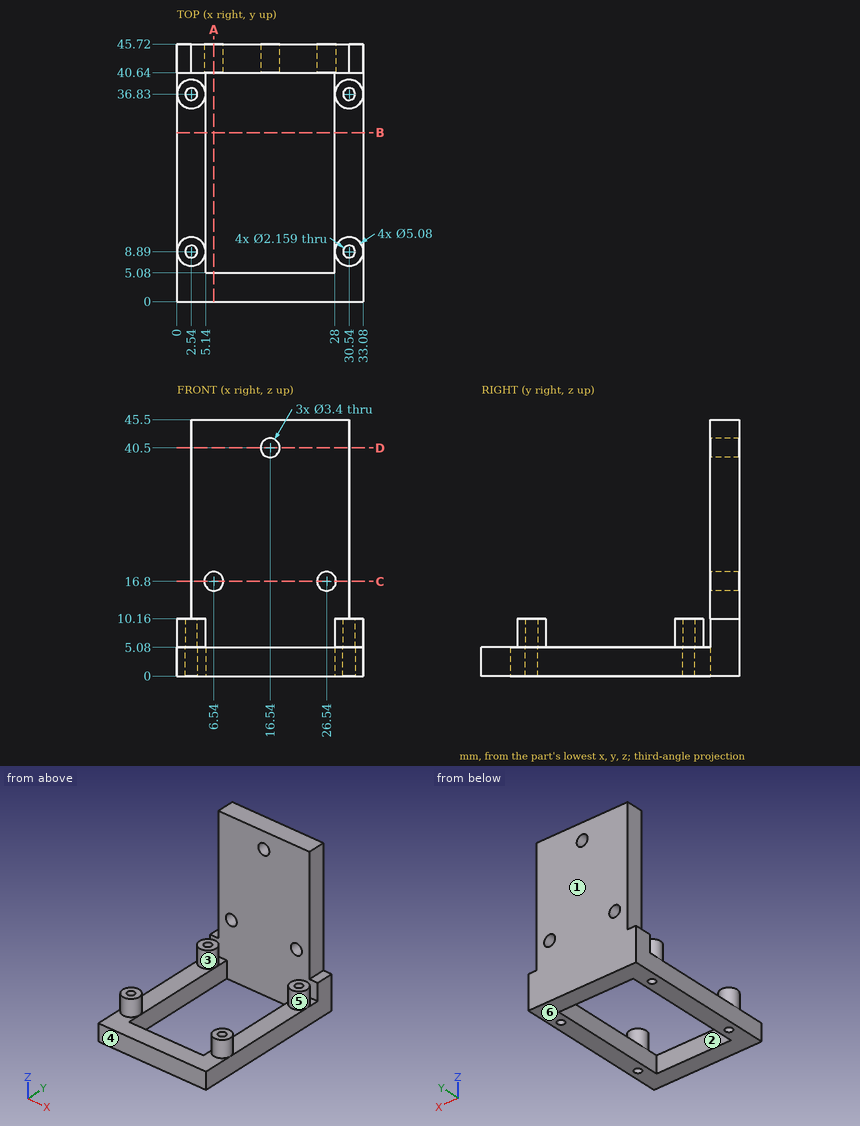
Could you check a few things on this drawing? It's one solid part, dimensions in mm from its lowest x, y, z. A direction names the side the tool comes from. Round coordinates to 2 decimals unless told otherwise and drop trailing zeros. Loops run counter-clockwise (first coordinate to the right, second up) from the corner with the lowest first, then second, coordinate; pieces in that order, holes last. Notation, with made-up numbers: (-24, 86) -> (15, 86) arc R10 ccw to (15, 90) -> close; hole circle Ø7 at (-17.75, -2.5). An arc over 180 degrees is marked (long way). Answer as CSV lines item,"result".
1. If we section it at D-D on z = 40.5: Please give me the cut outline in (x, y), plus the area to 3 significant figures.
Final values:
outline,"(2.54, 40.64) -> (14.84, 40.64) -> (14.84, 45.72) -> (2.54, 45.72) -> close; (18.24, 40.64) -> (30.54, 40.64) -> (30.54, 45.72) -> (18.24, 45.72) -> close"
area,"125 mm^2"
2. Thinking about a two-plate mould opening in Y: for the marked faces 4, 5 and 6, which applies, released by +Y, released by -Y, zero draft, split by the parting line, or undercut?
Final values:
face 4,"released by -Y"
face 5,"undercut"
face 6,"zero draft"
3. If we section it at B-B on y = 30: Please give me the cut outline in (x, z), plus the area to 3 significant figures.
Final values:
outline,"(0, 0) -> (5.14, 0) -> (5.14, 5.08) -> (0, 5.08) -> close; (28, 0) -> (33.08, 0) -> (33.08, 5.08) -> (28, 5.08) -> close"
area,"51.9 mm^2"
4. If I drill on L1, parallel to Y at x = 30.54, z = 7.35; L2, parallel to Y at x = 30.54, z = 3.3; L3, parallel to Y at x = 30, z = 1, over which ranges is the centre line in solid material (lowest first)?
Final values:
L1,"y = 6.35 to 7.81, 9.97 to 11.43, 34.29 to 35.75, 37.91 to 39.37, 40.64 to 45.72"
L2,"y = 0 to 7.81, 9.97 to 35.75, 37.91 to 45.72"
L3,"y = 0 to 7.96, 9.82 to 35.9, 37.76 to 45.72"
5. If we section it at A-A on x = 6.54: Please give me the cut outline in (y, z), plus the area to 3 significant figures.
Final values:
outline,"(0, 0) -> (5.08, 0) -> (5.08, 5.08) -> (0, 5.08) -> close; (40.64, 0) -> (45.72, 0) -> (45.72, 15.1) -> (40.64, 15.1) -> close; (40.64, 18.5) -> (45.72, 18.5) -> (45.72, 45.5) -> (40.64, 45.5) -> close"
area,"240 mm^2"
6. Which directions (+Z, -Z, +X, -X, +Y, -Y) give clear straight access to the entire face, cutting with the end or side of a thin tool? Please do the marked faces 1, 2 and 3.
Final values:
face 1,"+Z, -Z, +X, -X, +Y"
face 2,"+Z, -Z"
face 3,"+Z"
7. If we section it at C-C on z = 16.8: Please give me the cut outline in (x, y), plus the area to 3 significant figures.
Final values:
outline,"(2.54, 40.64) -> (4.84, 40.64) -> (4.84, 45.72) -> (2.54, 45.72) -> close; (8.24, 40.64) -> (24.84, 40.64) -> (24.84, 45.72) -> (8.24, 45.72) -> close; (28.24, 40.64) -> (30.54, 40.64) -> (30.54, 45.72) -> (28.24, 45.72) -> close"
area,"108 mm^2"
8. For pin 1 (1.3 mm diameter, centred on x = 1, y = 43.5, fed in from +Z); pin 2 (1 mm diameter, centred on x = 7.5, y = 35, fed in from -Z); pin 3 (5 mm diameter, centred on x = 17.5, z = 21.5, fed in from -Y), each with a flat end and sliding along its axis, tell me the tip position at first contact or that it passes through.
Final values:
pin 1,"stops at z = 10.16"
pin 2,"passes through"
pin 3,"stops at y = 40.64"
